Part model, mm, in its own coordinate system. Face numbers are marked on the shaded views. Round coordinates to 2 decimals unless told otherwise and drop trailing zeros. Loops run counter-clockwise (first coordinate to the right, second up) from the corner with the lowest first, then second, coordinate; pieces in that order, holes last. Notation, with made-up numbers: (46, -29.5) - (71, -29.5) arc R29 ccw to (71, -7.5) - close; hole circle Ø4 at (58.25, -2). An arc over 180 degrees is marked (long way). Put each result on its own line as item: value.
from build123d import *

# Parameters (mm, degrees)
SKETCH_2_R               = 10
EXTRUDE_2_DEPTH          = 2.5
EXTRUDE_3_DEPTH          = 47
EXTRUDE_4_DEPTH          = 47
CUT_EXTRUDE_2_DEPTH      = 45
EXTRUDE_5_DEPTH          = 4
EXTRUDE_6_DEPTH          = 49.5
EXTRUDE_6_DEPTH_BACK     = 20.5
SKETCH_5_R               = 35
SKETCH_5_R_2             = 7
EXTRUDE_8_DEPTH          = 24.5
EXTRUDE_8_DEPTH_BACK     = 5.5
SKETCH_6_3_R             = 23.5
SKETCH_6_3_R_2           = 7
CUT_EXTRUDE_START        = -3.861407426
CUT_EXTRUDE_4_OUTLINE_R  = 7
CUT_EXTRUDE_4_DEPTH      = 3.861407426
CUT_EXTRUDE_5_DEPTH      = 31
CUT_EXTRUDE_5_DEPTH_BACK = 118
SKETCH_10_R              = 6.5
CUT_EXTRUDE_7_DEPTH      = 10
SKETCH_13_R              = 23.5
SKETCH_13_R_2            = 7
EXTRUDE_9_DEPTH          = 5
SKETCH_14_R              = 7
CUT_EXTRUDE_8_DEPTH      = 326


# Read off the part's stored shape, not the designer's step: the extrude step
with BuildPart() as part:
    # Sketch 2 → Extrude 2 (new body)
    with BuildSketch(Plane(origin=(0, 0, 0), x_dir=(1, 0, 0), z_dir=(0, 1, 0))):
        with BuildLine():
            add(Edge.make_bspline(
                [(66.535337275, 366.960093359), (97.433190899, 191.906412215), (25.491327677, 30.335008843)],
                knots=[0, 0, 0, 1, 1, 1], degree=2))
            Line((25.491327677, 30.335008843), (298.070406458, 20.879087079))
            Line((298.070406458, 20.879087079), (381.06378597, 18))
            Line((381.06378597, 18), (480.018834564, 18))
            Line((480.018834564, 18), (480.018834564, 81))
            Line((480.018834564, 81), (403.59654847, 81))
            ThreePointArc((403.59654847, 81), (384.052422459, 84.272342385), (366.640132179, 93.732428718))
            Line((366.640132179, 93.732428718), (354.182306501, 103.472649748))
            Line((354.182306501, 103.472649748), (66.535337275, 366.960093359))
        make_face()
        with Locations(Location((63.069024618, 52.166207095, 0), (0, 0, 270))):
            Circle(SKETCH_2_R, mode=Mode.SUBTRACT)
        with BuildLine():
            Line((210.484938228, 194.417109435), (265.843761834, 143.707884329))
            Line((265.843761834, 143.707884329), (280.267263132, 130.495815747))
            ThreePointArc((280.267263132, 130.495815747), (290.530388989, 86.505736508), (253.248807869, 61.00000121))
            Line((253.248807869, 61.00000121), (167.295718615, 61.00000121))
            Line((167.295718615, 61.00000121), (119.992311174, 61.00000121))
            ThreePointArc((119.992311174, 61.00000121), (89.633225011, 74.955311015), (80.457661489, 107.083706844))
            Line((80.457661489, 107.083706844), (96.920664861, 214.067691653))
            ThreePointArc((96.920664861, 214.067691653), (123.181449566, 245.717320201), (163.47376981, 237.479800556))
            Line((163.47376981, 237.479800556), (210.484938228, 194.417109435))
        make_face(mode=Mode.SUBTRACT)
        with Locations(Location((323.151772468, 73.823254893, 0), (0, 0, 270))):
            Circle(SKETCH_2_R, mode=Mode.SUBTRACT)
        with Locations(Location((111.566817708, 278.73398761, 0), (0, 0, 270))):
            Circle(SKETCH_2_R, mode=Mode.SUBTRACT)
    extrude(amount=EXTRUDE_2_DEPTH)

    # Sketch 2_4 → Extrude 3 (add)
    with BuildSketch(Plane(origin=(0, 0, 0), x_dir=(1, 0, 0), z_dir=(0, 1, 0))):
        Polygon((0, 31.026794813), (0, 27.216911211), (380.994425705, 14), (480.018834564, 14), (480.018834564, 18), (381.06378597, 18), (298.070406458, 20.879087079), (25.491327677, 30.335008843), align=None)
        with BuildLine():
            ThreePointArc((50.999725499, 373), (59.333927702, 371.436909143), (66.535337275, 366.960093359))
            Line((66.535337275, 366.960093359), (354.182306501, 103.472649748))
            Line((354.182306501, 103.472649748), (366.640132179, 93.732428718))
            ThreePointArc((366.640132179, 93.732428718), (384.052422459, 84.272342385), (403.59654847, 81))
            Line((403.59654847, 81), (480.018834564, 81))
            Line((480.018834564, 81), (480.018834564, 85))
            Line((480.018834564, 85), (403.59654847, 85))
            ThreePointArc((403.59654847, 85), (385.355364193, 88.054186226), (369.103893265, 96.883600137))
            Line((369.103893265, 96.883600137), (356.892394312, 106.431229232))
            Line((356.892394312, 106.431229232), (356.884152027, 106.422231202))
            Line((356.884152027, 106.422231202), (356.769043373, 106.527671857))
            Line((356.769043373, 106.527671857), (68.090449936, 370.960093359))
            ThreePointArc((68.090449936, 370.960093359), (60.889040363, 375.436909143), (52.554838159, 377))
            Line((52.554838159, 377), (0, 377))
            Line((0, 377), (0, 373))
            Line((0, 373), (50.999725499, 373))
        make_face()
    extrude(amount=EXTRUDE_3_DEPTH)

    # Sketch 2_6 → Extrude 4 (add)
    with BuildSketch(Plane(origin=(0, 0, 0), x_dir=(1, 0, 0), z_dir=(0, 1, 0))):
        Polygon((0, 27.216911211), (0, 0), (480.018834564, 0), (480.018834564, 13.998527319), (480.018834564, 14), (380.994425705, 14), align=None)
        with BuildLine():
            Line((403.59654847, 85), (480.018834564, 85))
            Line((480.018834564, 85), (480.018834564, 115))
            Line((480.018834564, 115), (419.702060514, 115))
            ThreePointArc((419.702060514, 115), (397.96066346, 119.077628321), (379.174377619, 130.756278195))
            Line((379.174377619, 130.756278195), (91.527408393, 394.243721805))
            ThreePointArc((91.527408393, 394.243721805), (72.741122552, 405.922371679), (50.999725499, 410))
            Line((50.999725499, 410), (0, 410))
            Line((0, 410), (0, 377))
            Line((0, 377), (52.554838159, 377))
            ThreePointArc((52.554838159, 377), (60.889040363, 375.436909143), (68.090449936, 370.960093359))
            Line((68.090449936, 370.960093359), (356.769043373, 106.527671857))
            Line((356.769043373, 106.527671857), (369.103893265, 96.883600137))
            ThreePointArc((369.103893265, 96.883600137), (385.355364193, 88.054186226), (403.59654847, 85))
        make_face()
    extrude(amount=EXTRUDE_4_DEPTH)

    # Sketch 2_8 → Cut-Extrude 2 (cut)
    with BuildSketch(Plane(origin=(0, 0, 0), x_dir=(1, 0, 0), z_dir=(0, 1, 0))):
        Polygon((0, 27.216911211), (0, 0), (480.018834564, 0), (480.018834564, 13.998527319), (480.018834564, 14), (380.994425705, 14), (25.352648845, 26.337413543), align=None)
        with BuildLine():
            Line((403.59654847, 85), (480.018834564, 85))
            Line((480.018834564, 85), (480.018834564, 115))
            Line((480.018834564, 115), (419.702060514, 115))
            ThreePointArc((419.702060514, 115), (397.96066346, 119.077628321), (379.174377619, 130.756278195))
            Line((379.174377619, 130.756278195), (356.892394312, 106.431229232))
            Line((356.892394312, 106.431229232), (369.103893265, 96.883600137))
            ThreePointArc((369.103893265, 96.883600137), (385.355364193, 88.054186226), (403.59654847, 85))
        make_face()
        with BuildLine():
            Line((356.769043373, 106.527671857), (356.892394312, 106.431229232))
            Line((356.892394312, 106.431229232), (379.174377619, 130.756278195))
            Line((379.174377619, 130.756278195), (91.527408393, 394.243721805))
            ThreePointArc((91.527408393, 394.243721805), (72.741122552, 405.922371679), (50.999725499, 410))
            Line((50.999725499, 410), (50, 410))
            Line((50, 410), (0, 410))
            Line((0, 410), (0, 377))
            Line((0, 377), (4, 377))
            Line((4, 377), (52.554838159, 377))
            ThreePointArc((52.554838159, 377), (60.889040363, 375.436909143), (68.090449936, 370.960093359))
            Line((68.090449936, 370.960093359), (69.237182801, 369.909674812))
            Line((69.237182801, 369.909674812), (88.862343813, 351.93283494))
            Line((88.862343813, 351.93283494), (356.769043373, 106.527671857))
        make_face()
    extrude(amount=CUT_EXTRUDE_2_DEPTH, mode=Mode.SUBTRACT)

    # Sketch 3 → Extrude 5 (add)
    with BuildSketch(Plane(origin=(0, 47, 0), x_dir=(1, 0, 0), z_dir=(0, 1, 0))):
        with BuildLine():
            Line((295.056115028, 13.302883956), (405.018705009, 10.434294652))
            add(Edge.make_bspline(
                [(410.482503132, 81), (385.175508217, 49.842434065), (405.018705009, 10.434294652)],
                knots=[0.140921029, 0.140921029, 0.140921029, 1, 1, 1], degree=2))
            Line((410.482503132, 81), (403.59654847, 81))
            ThreePointArc((403.59654847, 81), (387.212309845, 83.280361014), (372.07347052, 89.948109177))
            add(Edge.make_bspline(
                [(372.07347052, 89.948109177), (362.166146879, 35.323611031), (295.056115028, 13.302883956)],
                knots=[0.241603801, 0.241603801, 0.241603801, 1, 1, 1], degree=2))
        make_face()
        with BuildLine():
            Line((403.59654847, 81), (410.482503132, 81))
            add(Edge.make_bspline(
                [(420, 91), (414.633795266, 86.111004243), (410.482503132, 81)],
                knots=[0, 0, 0, 0.140921029, 0.140921029, 0.140921029], degree=2))
            add(Edge.make_bspline(
                [(420, 91), (390.907181835, 102.66550813), (372.580466903, 128.060677104)],
                knots=[0, 0, 0, 1, 1, 1], degree=2))
            add(Edge.make_bspline(
                [(372.580466903, 128.060677104), (375.229666524, 107.349945336), (372.07347052, 89.948109177)],
                knots=[0, 0, 0, 0.241603801, 0.241603801, 0.241603801], degree=2))
            ThreePointArc((372.07347052, 89.948109177), (387.212309845, 83.280361014), (403.59654847, 81))
        make_face()
    extrude(amount=EXTRUDE_5_DEPTH)

    # Sketch 5 → Extrude 6 (add, two sides: drawn at the far end of the back side and taken through both)
    with BuildSketch(Plane(origin=(0, 0, -377), x_dir=(-1, 0, 0), z_dir=(0, 0, -1)).offset(-EXTRUDE_6_DEPTH_BACK)):
        with Locations((0, 22.5)):
            Circle(SKETCH_5_R)
        with Locations((0, 22.5)):
            Circle(SKETCH_5_R_2, mode=Mode.SUBTRACT)
    extrude(amount=EXTRUDE_6_DEPTH + EXTRUDE_6_DEPTH_BACK)

    # Sketch 6_3 → Extrude 8 (add, two sides: drawn at the far end of the back side and taken through both)
    with BuildSketch(Plane(origin=(0.943035097, 0, -27.184196792), x_dir=(0.9993988249637922, 0, 0.03466970811806164), z_dir=(-0.03466970811806164, 0, 0.9993988249637923)).offset(-EXTRUDE_8_DEPTH_BACK)):
        with Locations((-0.943602368, 22.5)):
            Circle(SKETCH_6_3_R)
        with Locations((-0.943602368, 22.5)):
            Circle(SKETCH_6_3_R_2, mode=Mode.SUBTRACT)
    extrude(amount=EXTRUDE_8_DEPTH + EXTRUDE_8_DEPTH_BACK)

    # Cut-Extrude 4 outline → Cut-Extrude 4 (cut)
    with BuildSketch(Plane(origin=(0.943035097, 0, -27.184196792), x_dir=(0.9993988249637922, 0, 0.03466970811806164), z_dir=(-0.03466970811806164, 0, 0.9993988249637923)).offset(CUT_EXTRUDE_START)):
        with Locations((-0.943602368, 22.5)):
            Circle(CUT_EXTRUDE_4_OUTLINE_R)
    extrude(amount=CUT_EXTRUDE_4_DEPTH, mode=Mode.SUBTRACT)

    # Sketch 10 → Cut-Extrude 5 (cut, two sides: drawn at the far end of the back side and taken through both)
    with BuildSketch(Plane(origin=(0, 0, -85), x_dir=(-1, 0, 0), z_dir=(0, 0, -1)).offset(-CUT_EXTRUDE_5_DEPTH_BACK)):
        with Locations(Location((-437.748834564, 28, 0), (0, 0, 180))):
            Circle(SKETCH_10_R)
    extrude(amount=CUT_EXTRUDE_5_DEPTH + CUT_EXTRUDE_5_DEPTH_BACK, mode=Mode.SUBTRACT)

    # Sketch 12 → Cut-Extrude 7 (cut)
    with BuildSketch(Plane(origin=(0, 47, 0), x_dir=(1, 0, 0), z_dir=(0, 1, 0))):
        Polygon((0, 0), (9.608777796, 0), (9.608777796, 2.511490201), (9.608777796, 2.911490201), (5, 2.911490201), (0, 2.911490201), (0, 2.3), align=None)
    extrude(amount=-CUT_EXTRUDE_7_DEPTH, mode=Mode.SUBTRACT)

    # Sketch 13 → Extrude 9 (add)
    with BuildSketch(Plane(origin=(0.093627248, 0, -2.698925581), x_dir=(0.9993988249637922, 0, 0.03466970811806163), z_dir=(-0.03466970811806163, 0, 0.9993988249637923))):
        with Locations((-0.943602368, 22.5)):
            Circle(SKETCH_13_R)
        with Locations((-0.943602368, 22.5)):
            Circle(SKETCH_13_R_2, mode=Mode.SUBTRACT)
    extrude(amount=-EXTRUDE_9_DEPTH)

    # Sketch 14 → Cut-Extrude 8 (cut)
    with BuildSketch(Plane(origin=(0, 0, -426.5), x_dir=(-1, 0, 0), z_dir=(0, 0, -1))):
        with Locations((0, 22.5)):
            Circle(SKETCH_14_R)
    extrude(amount=-CUT_EXTRUDE_8_DEPTH, mode=Mode.SUBTRACT)


solid = part.part
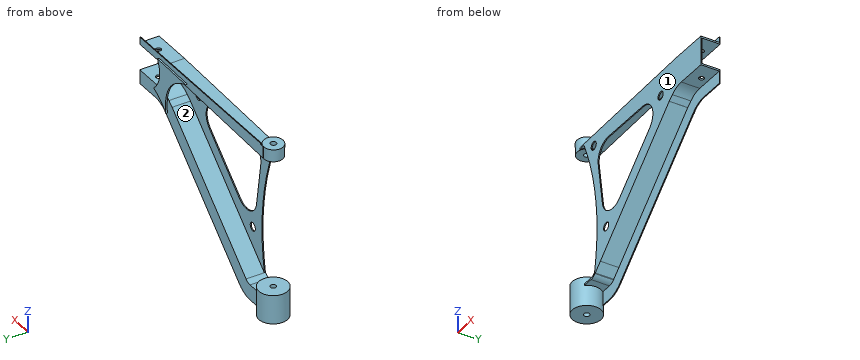
1. Two-plate mould, pull along Z, no slides. Class the marked faces 1 and 2: pulls with the +Z half, pulls with the -Z half, needs draft (parallel to the pull), parting line crosses it, or undercut.
A:
face 1: needs draft
face 2: undercut
2. Probe line 1 along Y through (x, z) = (77, -365.5); line 2 along Z through (x, y) = (377.5, 7); line 3 along Y through (x, z) = (81, -350). List the from-to ranges inside material, lowest first. Write a range as [from, to].
A:
line 1: y = [45, 47]
line 2: z = [-91.45, -86.97], [-18.12, -14.12]
line 3: y = [0, 2.5]
3. Band-saw the part on A-A (x = 144). List the corners of the cut face in (y, z).
A:
outline: (0, -301.43) - (45, -301.43) - (45, -346.18) - (47, -346.18) - (47, -296) - (2.5, -296) - (2.5, -247.27) - (0, -247.27) - close; (0, -61) - (2.5, -61) - (2.5, -26.22) - (47, -26.22) - (47, 0) - (45, 0) - (45, -22.22) - (0, -22.22) - close
4. Pin check, flat tips, straight feed: P1, Ø15, axis at x = 437.75, y = 28, coming from the -Z side; P2, Ø5, axis at y = 17, z = -359, coming from the -X side; P3, Ø0.6, axis at x = 6, y = 45.5, coming from the +Z side; P4, Ø11, axis at x = 0, y = 22.5, coming from the +Z side. Stop position of each tip, or through.
A:
P1: stops at z = -85
P2: stops at x = -34.87
P3: stops at z = -2.91
P4: passes through
